Geometry check sheet. Reference: drawing and pictorial views, mm from the part's lowest x, y, z. Give positions to 0.01 mm unless a question says otherwise; leave off trailing zeros. Order: outer loops, then holes, each group sorted by start corner. A loop starts at its lowest first (then second) coordinate and runs counter-clockwise, first axis right, second up.
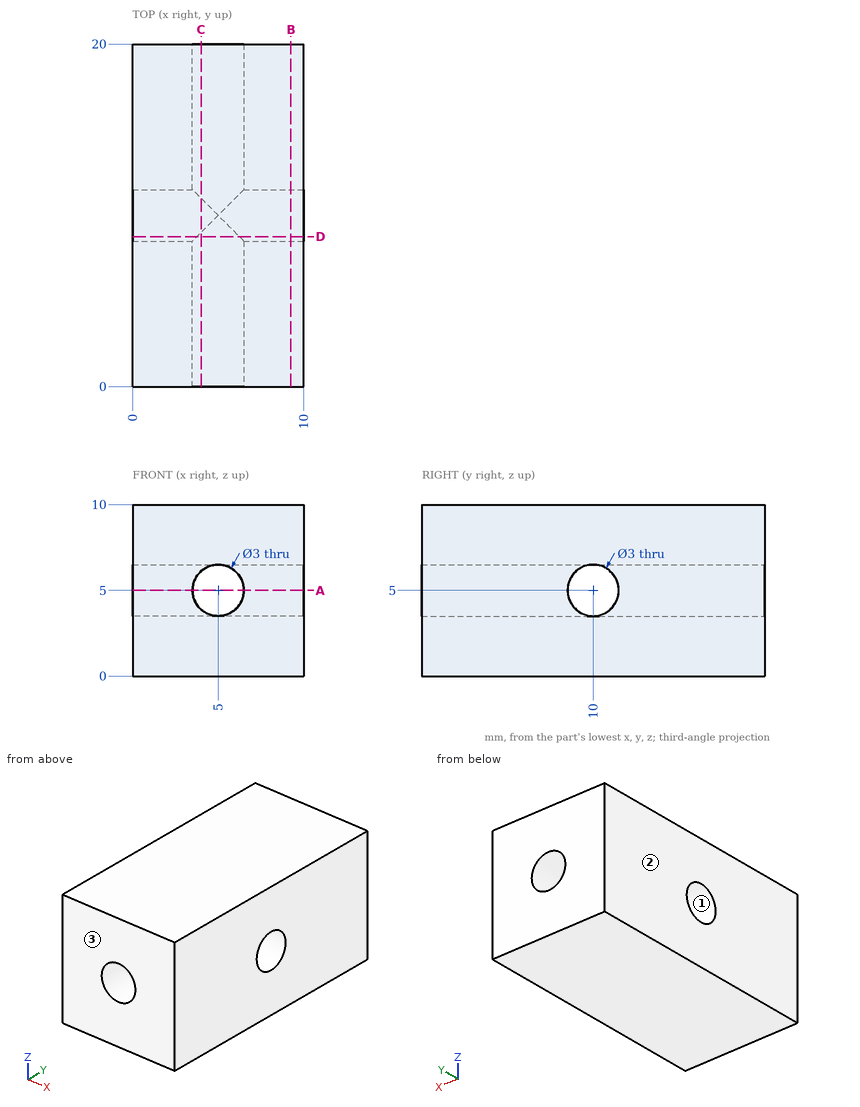
(1) Cross-section at A-A on z = 5. Enter the section's corners in (x, y), then the cut area to 3 significant figures.
Response values:
outline: (0, 0) - (3.5, 0) - (3.5, 8.5) - (0, 8.5) - close; (0, 11.5) - (3.5, 11.5) - (3.5, 20) - (0, 20) - close; (6.5, 0) - (10, 0) - (10, 8.5) - (6.5, 8.5) - close; (6.5, 11.5) - (10, 11.5) - (10, 20) - (6.5, 20) - close
area: 119 mm2
(2) Material ranges on L1, parallel to Y at x = 8.8, z = 5; L2, parallel to X at y = 5.75, z = 5, recorded low to high.
Response values:
L1: y = 0 to 8.5, 11.5 to 20
L2: x = 0 to 3.5, 6.5 to 10
(3) Release check for a two-part mould opening along Y. For the marked faces 1, 2 and 3 record: released by +Y, released by -Y, zero draft, split by the parting line, or undercut.
Response values:
face 1: undercut
face 2: zero draft
face 3: released by -Y
(4) Cross-section at D-D on y = 8.75. Enter the section's corners in (x, z), then the cut area to 3 significant figures.
Response values:
outline: (0, 0) - (10, 0) - (10, 4.17) - (6.25, 4.17) arc R1.5 cw to (3.75, 4.17) - (0, 4.17) - close; (0, 5.83) - (3.75, 5.83) arc R1.5 cw to (6.25, 5.83) - (10, 5.83) - (10, 10) - (0, 10) - close
area: 81.1 mm2
(5) Cross-section at C-C on x = 4. Enter the section's corners in (y, z), then the cut area to 3 significant figures.
Response values:
outline: (0, 0) - (20, 0) - (20, 3.88) - (11, 3.88) arc R1.5 cw to (9, 3.88) - (0, 3.88) - close; (0, 6.12) - (9, 6.12) arc R1.5 cw to (11, 6.12) - (20, 6.12) - (20, 10) - (0, 10) - close
area: 154 mm2
(6) Cross-section at B-B on x = 9.25. Enter the section's corners in (y, z).
Response values:
outline: (0, 0) - (20, 0) - (20, 10) - (0, 10) - close; hole circle Ø3 at (10, 5)
(7) Gauge pin test, flat end, axial feed: pin 1 Ø2.5 at (y, z) = (10, 5) entering from -X. Record the tip position at first contact, or that the pin passes through.
Response values:
pin 1: passes through
